from build123d import *

# Parameters (mm, degrees)
SKETCH1_W           = 58.9788
SKETCH1_H           = 41.275
BOSS_EXTRUDE1_DEPTH = 3.175
SKETCH2_W           = 12.7
SKETCH2_H           = 28.575
SKETCH2_W_2         = 33.5788
CUT_EXTRUDE1_DEPTH  = 37.133249835
FILLET1_R           = 2.54


with BuildPart() as part:
    # Sketch1 → Boss-Extrude1 (new body)
    with BuildSketch(Plane.XY):
        Rectangle(SKETCH1_W, SKETCH1_H)
    extrude(amount=BOSS_EXTRUDE1_DEPTH)

    # Sketch2 → Cut-Extrude1 (cut, through all)
    with BuildSketch(Plane.XY.offset(3.175)):
        with Locations((23.1394, 0)):
            Rectangle(SKETCH2_W, SKETCH2_H)
        with Locations((-6.35, 0)):
            Rectangle(SKETCH2_W_2, SKETCH2_H)
    extrude(amount=-CUT_EXTRUDE1_DEPTH, mode=Mode.SUBTRACT)

    # Fillet1
    fillet1_edges = [part.edges().sort_by_distance(p)[0] for p in [
        (16.7894, -14.2875, 1.5875),
        (16.7894, 14.2875, 1.5875),
        (10.4394, 14.2875, 1.5875),
        (10.4394, -14.2875, 1.5875),
        (-23.1394, -14.2875, 1.5875),
        (-23.1394, 14.2875, 1.5875),
    ]]
    fillet(fillet1_edges, radius=FILLET1_R)


solid = part.part
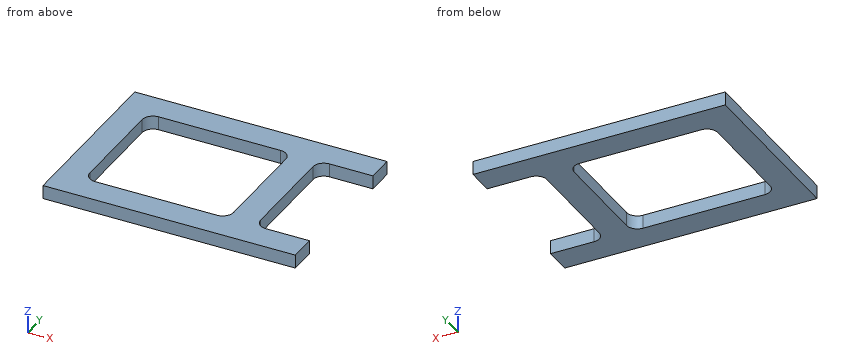
Design review of the part built by this model. Coordinates are the model's own, in mm. Round coordinates to 2 decimals unless told otherwise and drop trailing zeros. Write each loop counter-clockwise with the first axis right and the second up, starting at its lowest first coordinate (ties: lowest second). Pieces come first, ordered by that corner, then holes. Notation, with made-up numbers: (16, 9) - (57, 9) arc R31 cw to (57, 46) - close; hole circle Ø2 at (79.5, 40.25). An arc over 180 degrees is marked (long way). Use a Markdown table: item, result. Add a question column.
1. Clearance check with a flat-ended pin moving along its axis: pin 1 (10 mm diameter, centred on x = -19.5, y = 10.5, fed in from -Z). State where the tip first meets the part, or that it passes through.
2. We need section A-A (y = 10). State the section outline as (x, z) points (3 decimals).
3. We need section B-B (x = -18.5). State the section outline as (y, z) points (1 decimal).
4. Wall thickness on probe 1 along Y at (x, z) = (0.5, 0.4); probe 2 along X at (y, z) = (7, 2.65); probe 3 along X at (y, z) = (-13, 0.95): over which ranges is each line inside the solid? List them lowest first.
5. We need section C-C (z = 1.4). State the section outline as (x, y) points.
Output:
| question | item | result |
|---|---|---|
| 1 | pin 1 | stops at z = 0 |
| 2 | outline | (-29.489, 0) - (-23.139, 0) - (-23.139, 3.175) - (-29.489, 3.175) - close; (10.439, 0) - (16.789, 0) - (16.789, 3.175) - (10.439, 3.175) - close |
| 3 | outline | (-20.6, 0) - (-14.3, 0) - (-14.3, 3.2) - (-20.6, 3.2) - close; (14.3, 0) - (20.6, 0) - (20.6, 3.2) - (14.3, 3.2) - close |
| 4 | probe 1 | y = -20.64 to -14.29, 14.29 to 20.64 |
| 4 | probe 2 | x = -29.49 to -23.14, 10.44 to 16.79 |
| 4 | probe 3 | x = -29.49 to -22.81, 10.11 to 17.12 |
| 5 | outline | (-29.49, -20.64) - (29.49, -20.64) - (29.49, -14.29) - (19.33, -14.29) arc R2.54 cw to (16.79, -11.75) - (16.79, 11.75) arc R2.54 cw to (19.33, 14.29) - (29.49, 14.29) - (29.49, 20.64) - (-29.49, 20.64) - close; hole (-23.14, -11.75) arc R2.54 ccw to (-20.6, -14.29) - (7.9, -14.29) arc R2.54 ccw to (10.44, -11.75) - (10.44, 11.75) arc R2.54 ccw to (7.9, 14.29) - (-20.6, 14.29) arc R2.54 ccw to (-23.14, 11.75) - close |
